The listing builds one solid part. Answer for the finished solid, in the listing's coordinates (mm). A direction names the side the tool comes from. Round coordinates to 2 decimals unless told otherwise and drop trailing zeros. Write each loop counter-clockwise with the first axis right and the second up, starting at its lowest first coordinate (ties: lowest second). Pieces come first, ordered by that corner, then holes. Notation, with made-up numbers: (26.25, 68) - (56.25, 68) arc R28 ccw to (56.25, 98) - close; hole circle Ø6 at (-4, 78). An arc over 180 degrees is marked (long way). Use a Markdown table: item, result. Add a question column.
1) Find the intervals of material crossed by probe 1 along X at (y, z) = (10, 6.25); probe 2 along X at (y, z) = (26.5, 9.75), in increasing order. Write a range as from..to.
2) A cutting plane is placed at B-B (z = 11.5). Give the vertices of the cut face in (x, y).
3) Determine the mould class of faces 4 (the cylindrical face through (4.57, 4.6, 8.11)), 5 (the cylindrical face through (15.715, 15.699, 8.112)), 6 (the flat face through (3, 13, 16)), 7 (the flat face through (12, 10, 8)) for opening direction X: +X half, -X half, draft (parallel to the pull), parting line (faces both ways), or undercut.
4) A cutting plane is placed at C-C (y = 28.5). Give the vertices of the cut face in (x, z).
5) Each of these flat-tipped pins is pushed along its axis until it touches: P1, Ø1, axis at x = 12.5, y = 14.5, coming from the -Z side; P2, Ø0.6, axis at x = 13.5, z = 12, coming from the +Y side; P3, Ø2, axis at x = 7.5, z = 9, coming from the +Y side. Where does it stop, or does it pass through?
6) A cutting plane is placed at A-A (y = 15.5). Give the vertices of the cut face in (x, z), then the cut area to 3 significant figures.
7) A tool of negligible diameter and unlimited length cuts with its end or side. For faces 1 (the flat face through (2, 32, 8)), 2 (the cylindrical face through (12.301, 15.715, 8.112)), 3 (the flat face through (14, 16, 8)), from which of +Z, -Z, +X, -X, +Y, -Y can it reach the whole face along a straight path? Write none if from no direction.
```python
from build123d import *

# Parameters (mm, degrees)
PAD_DEPTH   = 16
FILLET_R    = 2
FILLET001_R = 2
FILLET002_R = 2
FILLET003_R = 2
FILLET004_R = 1
FILLET005_R = 1
FILLET006_R = 1
FILLET007_R = 1


with BuildPart() as part:
    # Sketch → Pad (new body)
    with BuildSketch(Plane.XY):
        Polygon((0, 0), (0, 32), (4, 32), (4, 4), (12, 4), (12, 16), (16, 16), (16, 0), align=None)
    extrude(amount=PAD_DEPTH)

    # Fillet
    fillet_edges = [part.edges().sort_by_distance(p)[0] for p in [
        (4, 4, 8),
    ]]
    fillet(fillet_edges, radius=FILLET_R)

    # Fillet001
    fillet001_edges = [part.edges().sort_by_distance(p)[0] for p in [
        (12, 4, 8),
    ]]
    fillet(fillet001_edges, radius=FILLET001_R)

    # Fillet002
    fillet002_edges = [part.edges().sort_by_distance(p)[0] for p in [
        (16, 0, 8),
    ]]
    fillet(fillet002_edges, radius=FILLET002_R)

    # Fillet003
    fillet003_edges = [part.edges().sort_by_distance(p)[0] for p in [
        (0, 0, 8),
    ]]
    fillet(fillet003_edges, radius=FILLET003_R)

    # Fillet004
    fillet004_edges = [part.edges().sort_by_distance(p)[0] for p in [
        (16, 16, 8),
    ]]
    fillet(fillet004_edges, radius=FILLET004_R)

    # Fillet005
    fillet005_edges = [part.edges().sort_by_distance(p)[0] for p in [
        (12, 16, 8),
    ]]
    fillet(fillet005_edges, radius=FILLET005_R)

    # Fillet006
    fillet006_edges = [part.edges().sort_by_distance(p)[0] for p in [
        (4, 32, 8),
    ]]
    fillet(fillet006_edges, radius=FILLET006_R)

    # Fillet007
    fillet007_edges = [part.edges().sort_by_distance(p)[0] for p in [
        (0, 32, 8),
    ]]
    fillet(fillet007_edges, radius=FILLET007_R)


solid = part.part
```
Entries:
| question | item | result |
|---|---|---|
| 1 | probe 1 | x = 0..4, 12..16 |
| 1 | probe 2 | x = 0..4 |
| 2 | outline | (0, 2) arc R2 ccw to (2, 0) - (14, 0) arc R2 ccw to (16, 2) - (16, 15) arc R1 ccw to (15, 16) - (13, 16) arc R1 ccw to (12, 15) - (12, 6) arc R2 cw to (10, 4) - (6, 4) arc R2 cw to (4, 6) - (4, 31) arc R1 ccw to (3, 32) - (1, 32) arc R1 ccw to (0, 31) - close |
| 3 | face 4 | undercut |
| 3 | face 5 | +X half |
| 3 | face 6 | draft |
| 3 | face 7 | undercut |
| 4 | outline | (0, 0) - (4, 0) - (4, 16) - (0, 16) - close |
| 5 | P1 | stops at z = 0 |
| 5 | P2 | stops at y = 16 |
| 5 | P3 | stops at y = 4 |
| 6 | outline | (0, 0) - (4, 0) - (4, 16) - (0, 16) - close; (12.13, 0) - (15.87, 0) - (15.87, 16) - (12.13, 16) - close |
| 6 | area | 124 mm² |
| 7 | face 1 | +Z, -Z, +X, -X, +Y |
| 7 | face 2 | +Z, -Z, +Y |
| 7 | face 3 | +Z, -Z, +X, +Y |
